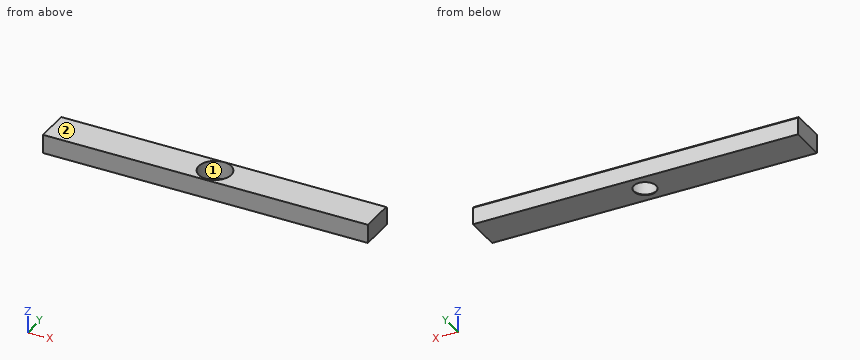
```python
from build123d import *

# Parameters (mm, degrees)
SKETCH1_W           = 950
SKETCH1_H           = 105
BOSS_EXTRUDE1_DEPTH = 27.5
SKETCH2_R           = 47.5
CUT_EXTRUDE1_DEPTH  = 53
SKETCH3_R           = 32.5
CUT_EXTRUDE2_DEPTH  = 481.822472437
CHAMFER1_SIZE       = 5


with BuildPart() as part:
    # Sketch1 → Boss-Extrude1 (new, symmetric)
    with BuildSketch(Plane.XY):
        Rectangle(SKETCH1_W, SKETCH1_H)
    extrude(amount=BOSS_EXTRUDE1_DEPTH, both=True)

    # Sketch2 → Cut-Extrude1 (cut)
    with BuildSketch(Plane.XY.offset(27.5)):
        Circle(SKETCH2_R)
    extrude(amount=-CUT_EXTRUDE1_DEPTH, mode=Mode.SUBTRACT)

    # Sketch3 → Cut-Extrude2 (cut, through all)
    with BuildSketch(Plane.XY.offset(-25.5)):
        Circle(SKETCH3_R)
    extrude(amount=-CUT_EXTRUDE2_DEPTH, mode=Mode.SUBTRACT)

    # Chamfer1
    chamfer1_edges = [part.edges().sort_by_distance(p)[0] for p in [
        (0, 52.5, 27.5),
    ]]
    chamfer(chamfer1_edges, length=CHAMFER1_SIZE - 0.0001)  # a hair under: the kernel refuses the full size


solid = part.part
```
Design review of the part built by this model. Coordinates are the model's own, in mm. Face numbers are marked on the shaded views. Coordinates: 2 decimals unless noted, no trailing zeros. Loops run counter-clockwise (first coordinate to the right, second up) from the corner with the lowest first, then second, coordinate; pieces in that order, holes last. Notation, with made-up numbers: (37, 7.5) - (50, 7.5) arc R15 cw to (50, 15.5) - close; hole circle Ø11 at (23.25, 55.25). An arc over 180 degrees is marked (long way). Use CSV: the item, a comma, the result in double quotes. Start each with the question number.
1) The part is to be moulded in two halves that separate along X. For the marked faces 1 and 2, say which applies: +X half, -X half, draft (parallel to the pull), parting line (faces both ways), or undercut.
2) Wall thickness on L1, parallel to Y at x = 0, z = 12; L2, parallel to Y at x = 0, z = -26; L3, parallel to Z at x = 19, y = -37: over which ranges is each line inside the solid? List them lowest first. Write a range as from..to.
3) Consider section A-A on y = 0. Write out the cut boundary in (x, z), then the cut area to 3 significant figures.
4) Consider section C-C on z = -8.5. Write out the cut boundary in (x, y), then the cut area to 3 significant figures.
Geometry says:
1,face 1,"undercut"
1,face 2,"draft"
2,L1,"-52.5..-47.5, 47.5..52.5"
2,L2,"-52.5..-32.5, 32.5..52.5"
2,L3,"-27.5..-25.5"
3,outline,"(-475, -27.5) - (-32.5, -27.5) - (-32.5, -25.5) - (-47.5, -25.5) - (-47.5, 27.5) - (-475, 27.5) - close; (32.5, -27.5) - (475, -27.5) - (475, 27.5) - (47.5, 27.5) - (47.5, -25.5) - (32.5, -25.5) - close"
3,area,"47,100 mm^2"
4,outline,"(-475, -52.5) - (475, -52.5) - (475, 52.5) - (-475, 52.5) - close; hole circle Ø95 at (0, 0)"
4,area,"92,700 mm^2"
